The listing builds one solid part. Answer for the finished solid, in the listing's coordinates (mm). Face numbers are marked on the shaded views. A direction names the side the tool comes from. Give positions to 0.01 mm unless a question says otherwise; leave off trailing zeros. Order: outer loops, then holes, each group sorted by start corner. A loop starts at its lowest first (then second) coordinate and runs counter-clockwise, first axis right, second up. Notation, with made-up numbers: (66.5, 53.5) - (92.5, 53.5) arc R17 cw to (92.5, 79.5) - close; hole circle Ø1 at (50, 41). An arc over 180 degrees is marked (long way). Use a Markdown table: item, result. Add a question column.
1) Straight lines are drawn through the part: line 1 (X direction, y = 2.25, z = -2); line 2 (X direction, y = 0.75, z = -2); line 3 (X direction, y = 2, z = -6.5). For each, find the intervals that lie inside material, in ascending order.
2) For the marked faces 5 and 6, determine the directions among +Z, -Z, +X, -X, +Y, -Y from which every point of the face is accessible in a straight line to the end or side of a thin tool.
3) Flat-ended cylindrical pins translate along their axes: pin 1 (3.5 mm diameter, centred on x = -8.5, z = -0.5, fed in from +Y); pin 2 (1.6 mm diameter, centred on x = 26.94, z = -2.57, fed in from +Y); pin 3 (4 mm diameter, centred on x = 37.94, z = -0.62, fed in from +Y). Find the tip coordinate at first contact, or state that the pin passes through.
4) The mould has two halves that part along Z. Classify the marked faces 1, 2, 3 and 4: released by +Z, released by -Z, zero draft, split by the parting line, or undercut.
5) Find section C-C, the plane y = 10.5. Determine the outline of the cut face in (x, z).
6) Find section B-B, the plane x = 9. Determine the outline of the cut face in (y, z), plus the area to 3 significant figures.
7) Find section A-A, the plane y = 2.2. Determine the outline of the cut face in (x, z).
from build123d import *

# Parameters (mm, degrees)
SKETCH1_W                 = 60
SKETCH1_H                 = 15
BOSS_EXTRUDE1_DEPTH       = 13
M2X0_4_TAPPED_HOLE1_D     = 1.6
CUT_EXTRUDE1_DEPTH        = 46.591613279
M6X1_0_TAPPED_HOLE1_D     = 5
M6X1_0_TAPPED_HOLE1_DEPTH = 10
M6X1_0_TAPPED_HOLE1_TIP   = 1.502151548
SKETCH15_R                = 3
CUT_EXTRUDE2_DEPTH        = 46.591613308
SKETCH16_R                = 5.5
CUT_EXTRUDE3_DEPTH        = 6.2


# Read off the part's stored shape, not the designer's step: M2x0.4 Tapped Hole2
with BuildPart() as part:
    # Sketch1 → Boss-Extrude1 (new body)
    with BuildSketch(Plane(origin=(0, 0, 0), x_dir=(1, 0, 0), z_dir=(0, 1, 0))):
        with Locations((12.93814433, 0.618556701)):
            Rectangle(SKETCH1_W, SKETCH1_H)
    extrude(amount=BOSS_EXTRUDE1_DEPTH)

    # M2x0.4 Tapped Hole1 (through all)
    with Locations(Plane(origin=(0, 0, -8.118556701), x_dir=(-1, 0, 0), z_dir=(0, 0, -1))):
        with Locations((-40.93814433, 2.2), (-8.93814433, 2.2)):
            Hole(M2X0_4_TAPPED_HOLE1_D / 2)

    # Sketch5 → Cut-Extrude1 (cut, through all)
    with BuildSketch(Plane(origin=(0, 13, 0), x_dir=(1, 0, 0), z_dir=(0, 1, 0))):
        with BuildLine():
            ThreePointArc((28.631734073, 1.585124743), (28.317002553, 1.997414924), (27.904712372, 2.312146445))
            ThreePointArc((27.904712372, 2.312146445), (26.93814433, 3.568556701), (25.971576288, 2.312146445))
            ThreePointArc((25.971576288, 2.312146445), (25.559286107, -0.760301522), (28.631734073, -0.348011341))
            ThreePointArc((28.631734073, -0.348011341), (29.88814433, 0.618556701), (28.631734073, 1.585124743))
        make_face()
    extrude(amount=-CUT_EXTRUDE1_DEPTH, mode=Mode.SUBTRACT)

    # M2x0.4 Tapped Hole2 outline → M2x0.4 Tapped Hole2 (revolve, cut)
    with BuildSketch(Plane(origin=(26.93814433, 6.5, 0), x_dir=(1, 0, 0), z_dir=(0, -1, 0))):
        Polygon((0, 1.227710243), (0.627359351, 1.227710243), (0.8, 1.331443299), (0.8, 6.881443299), (0, 6.881443299), align=None)
    revolve(axis=Axis((26.93814433, 6.5, 0), (0, 0, 1)), mode=Mode.SUBTRACT)

    # M6x1.0 Tapped Hole1
    with Locations(Plane(origin=(0, 13, 0), x_dir=(1, 0, 0), z_dir=(0, 1, 0))):
        with Locations((37.93814433, 0.618556701)):
            Hole(M6X1_0_TAPPED_HOLE1_D / 2, depth=M6X1_0_TAPPED_HOLE1_DEPTH)
            with Locations((0, 0, -(M6X1_0_TAPPED_HOLE1_DEPTH + M6X1_0_TAPPED_HOLE1_TIP / 2))):  # 118° drill point
                Cone(0, M6X1_0_TAPPED_HOLE1_D / 2, M6X1_0_TAPPED_HOLE1_TIP, mode=Mode.SUBTRACT)

    # Sketch15 → Cut-Extrude2 (cut, through all)
    with BuildSketch(Plane(origin=(0, 13, 0), x_dir=(1, 0, 0), z_dir=(0, 1, 0))):
        with Locations(Location((-11.06185567, 0.618556701, 0), (0, 0, 270))):
            Circle(SKETCH15_R)
        with Locations(Location((13.93814433, 0.618556701, 0), (0, 0, 270))):
            Circle(SKETCH15_R)
    extrude(amount=-CUT_EXTRUDE2_DEPTH, mode=Mode.SUBTRACT)

    # Sketch16 → Cut-Extrude3 (cut)
    with BuildSketch(Plane(origin=(0, 13, 0), x_dir=(1, 0, 0), z_dir=(0, 1, 0))):
        with Locations(Location((-11.06185567, 0.618556701, 0), (0, 0, 270))):
            Circle(SKETCH16_R)
        with Locations(Location((13.93814433, 0.618556701, 0), (0, 0, 270))):
            Circle(SKETCH16_R)
    extrude(amount=-CUT_EXTRUDE3_DEPTH, mode=Mode.SUBTRACT)


solid = part.part
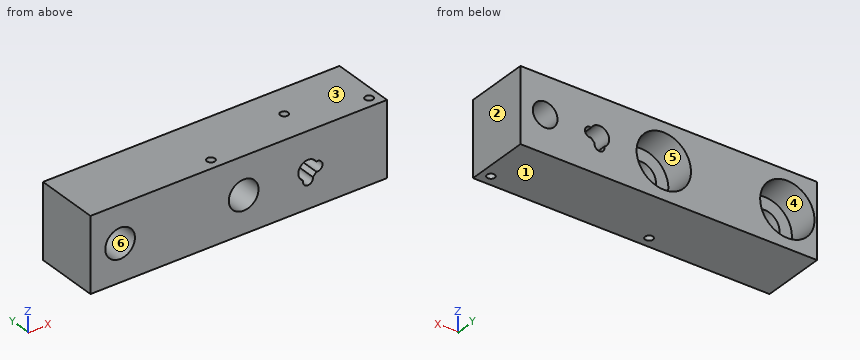
The answers:
| question | item | result |
|---|---|---|
| 1 | line 1 | -17.06 to -13.72, -8.4 to 8.14, 9.74 to 11.28, 16.6 to 25.56, 28.31 to 40.14, 41.74 to 42.94 |
| 1 | line 2 | -17.06 to -13.72, -8.4 to 11.28, 16.6 to 25.56, 28.31 to 42.94 |
| 1 | line 3 | -17.06 to 8.16, 9.71 to 40.16, 41.71 to 42.94 |
| 2 | face 5 | +Y |
| 2 | face 6 | +Y, -Y |
| 3 | pin 1 | y = 6.8 |
| 3 | pin 2 | through |
| 3 | pin 3 | y = 2.7 |
| 4 | face 1 | released by -Z |
| 4 | face 2 | zero draft |
| 4 | face 3 | released by +Z |
| 4 | face 4 | undercut |
| 5 | outline | (-17.06, -8.12) - (42.94, -8.12) - (42.94, 6.88) - (-17.06, 6.88) - close; hole circle Ø11 at (-11.06, -0.62); hole circle Ø11 at (13.94, -0.62); hole (25.97, -2.31) arc R1 ccw (long way) to (27.9, -2.31) arc R1.95 ccw to (28.63, -1.59) arc R1 ccw (long way) to (28.63, 0.35) arc R1.95 ccw (long way) to start; hole circle Ø5 at (37.94, -0.62) |
| 6 | outline | (0, -8.12) - (1.4, -8.12) - (1.4, 6.88) - (0, 6.88) - close; (3, -8.12) - (13, -8.12) - (13, -3.04) - (6.8, -3.04) - (6.8, 1.8) - (13, 1.8) - (13, 6.88) - (3, 6.88) - close |
| 6 | area | 141 mm2 |
| 7 | outline | (-17.06, -8.12) - (8.14, -8.12) - (8.14, 6.88) - (-17.06, 6.88) - close; (9.74, -8.12) - (40.14, -8.12) - (40.14, 6.88) - (9.74, 6.88) - close; (41.74, -8.12) - (42.94, -8.12) - (42.94, 6.88) - (41.74, 6.88) - close; hole circle Ø6 at (-11.06, -0.62); hole circle Ø6 at (13.94, -0.62); hole (25.97, -2.31) arc R1 ccw (long way) to (27.9, -2.31) arc R1.95 ccw to (28.63, -1.59) arc R1 ccw (long way) to (28.63, 0.35) arc R1.95 ccw (long way) to start; hole circle Ø2.34 at (37.94, -0.62) |
